```python
from build123d import *
from build123d.topology import SkipClean

# Parameters (mm, degrees)
BOSS_EXTRUDE1_DEPTH   = 20
CUT_EXTRUDE1_DEPTH    = 18.4
SKETCH3_W             = 14.5
SKETCH3_H             = 2.85
CUT_EXTRUDE2_DEPTH    = 18.4
SKETCH4_W             = 13
SKETCH4_H             = 1.4
BOSS_EXTRUDE2_DEPTH   = 22
BOSS_EXTRUDE2_2_DEPTH = 22
SKETCH5_W             = 13
SKETCH5_H             = 3.4
BOSS_EXTRUDE3_DEPTH   = 4
FILLET1_R             = 3.2
FILLET2_R             = 3.2
BOSS_EXTRUDE4_DEPTH   = 13
SKETCH8_W             = 0.8
SKETCH8_H             = 3.26
CUT_EXTRUDE3_DEPTH    = 13
FILLET3_R             = 3.2
FILLET4_R             = 0.8
SKETCH9_W             = 56.2
SKETCH9_H             = 1.6
BOSS_EXTRUDE5_DEPTH   = 10
SKETCH13_W            = 15.95
SKETCH13_H            = 1.6
CUT_EXTRUDE6_DEPTH    = 2
BOSS_EXTRUDE6_DEPTH   = 18.4
CUT_EXTRUDE5_START    = -18.4
SKETCH12_R            = 1.1
CUT_EXTRUDE5_DEPTH    = 18.4
SKETCH14_W            = 15.95
SKETCH14_H            = 5.75
CUT_EXTRUDE7_DEPTH    = 10


with BuildPart() as part:
    # Sketch1 → Boss-Extrude1 (new body)
    with BuildSketch(Plane(origin=(0, 0, 0), x_dir=(1, 0, 0), z_dir=(0, 1, 0))):
        Polygon((-38.4, 43.8), (-38.4, 40.4), (-21, 40.4), (-21, 43.8), (0, 43.8), (0, 0), (-21, 0), (-21, 3.4), (-38.4, 3.4), (-38.4, 0), (-59.4, 0), (-59.4, 43.8), align=None)
    extrude(amount=BOSS_EXTRUDE1_DEPTH)

    # Sketch2 → Cut-Extrude1 (cut)
    with BuildSketch(Plane(origin=(0, 20, 0), x_dir=(1, 0, 0), z_dir=(0, 1, 0))):
        Polygon((-57.8, 42.2), (-39.6, 42.2), (-39.6, 39.2), (-19.8, 39.2), (-19.8, 42.2), (-1.6, 42.2), (-1.6, 1.6), (-19.8, 1.6), (-19.8, 4.6), (-39.6, 4.6), (-39.6, 1.6), (-57.8, 1.6), align=None)
    extrude(amount=-CUT_EXTRUDE1_DEPTH, mode=Mode.SUBTRACT)

    # Sketch3 → Cut-Extrude2 (cut)
    with BuildSketch(Plane(origin=(0, 1.6, 0), x_dir=(1, 0, 0), z_dir=(0, 1, 0))):
        with Locations((-8.85, 37.875)):
            Rectangle(SKETCH3_W, SKETCH3_H)
    extrude(amount=-CUT_EXTRUDE2_DEPTH, mode=Mode.SUBTRACT)



with BuildPart() as body_2:
    # Sketch4 → Boss-Extrude2 (new body)
    with BuildSketch(Plane.XZ):
        with Locations((-29.7, -0.7)):
            Rectangle(SKETCH4_W, SKETCH4_H)
    extrude(amount=-BOSS_EXTRUDE2_DEPTH)


with BuildPart() as body_3:
    # Sketch4 → Boss-Extrude2 2 (new body)
    with BuildSketch(Plane.XZ):
        with Locations((-29.7, -43.1)):
            Rectangle(SKETCH4_W, SKETCH4_H)
    extrude(amount=-BOSS_EXTRUDE2_2_DEPTH)


with BuildPart() as part_1:
    add(part.part)

    add(body_2.part)  # Boss-Extrude3 merges body 2

    add(body_3.part)  # Boss-Extrude3 merges body 3
    # Sketch5 → Boss-Extrude3 (add)
    with BuildSketch(Plane(origin=(0, 0, 0), x_dir=(-1, 0, 0), z_dir=(0, -1, 0))):
        with Locations((29.7, 1.7)):
            Rectangle(SKETCH5_W, SKETCH5_H)
        with Locations((29.7, 42.1)):
            Rectangle(SKETCH5_W, SKETCH5_H)
    extrude(amount=-BOSS_EXTRUDE3_DEPTH)

    # Fillet1
    fillet1_edges = [part_1.edges().sort_by_distance(p)[0] for p in [
        (-29.7, 0, -43.8),
        (-29.7, 0, 0),
    ]]
    fillet(fillet1_edges, radius=FILLET1_R)

    # Fillet2
    # the kernel refuses this fillet: 3.2 mm, written as the material it adds along each edge
    with BuildSketch(Plane(origin=(-36.2, 4, -1.4), x_dir=(0, 0, -1), z_dir=(1, 0, 0)), Plane(origin=(-23.2, 4, -42.4), x_dir=(0, 0, 1), z_dir=(-1, 0, 0))) as fillet2_piece_1:
        with BuildLine():
            CenterArc((3.2, 2.966479395), FILLET2_R, 180, 67.975687163)
            Line((0, 2.966479395), (-0.064, 2.966479395))
            Line((-0.064, 2.966479395), (-0.064, 0))
            Line((-0.064, 0), (0, -0.064))
            ThreePointArc((0, -0.064), (1, -0.064), (1.976, -0.059329588))
            Line((1.976, -0.059329588), (2, 0))
        make_face()
    extrude(amount=13)

    # Sketch7 → Boss-Extrude4 (add)
    with BuildSketch(Plane(origin=(-23.2, 0, 0), x_dir=(0, 0, -1), z_dir=(1, 0, 0))):
        Polygon((-1.2, 17), (0, 17), (0, 11.8), align=None)
        Polygon((43.8, 11.8), (43.8, 17), (45, 17), align=None)
        Polygon((0, 22), (-3, 22), (-3, 20.26), (1.4, 20.26), (1.4, 22), (1.4, 26), (0, 26), align=None)
        Polygon((43.8, 22), (46.8, 22), (46.8, 20.26), (42.4, 20.26), (42.4, 22), (42.4, 26), (43.8, 26), align=None)
    extrude(amount=-BOSS_EXTRUDE4_DEPTH)

    # Sketch8 → Cut-Extrude3 (cut)
    with BuildSketch(Plane(origin=(-23.2, 0, 0), x_dir=(0, 0, -1), z_dir=(1, 0, 0))):
        with Locations((0.4, 18.63)):
            Rectangle(SKETCH8_W, SKETCH8_H)
        with Locations((43.4, 18.63)):
            Rectangle(SKETCH8_W, SKETCH8_H)
    extrude(amount=-CUT_EXTRUDE3_DEPTH, mode=Mode.SUBTRACT)

    # Fillet3
    # the kernel refuses this fillet: 3.2 mm, written as the material it adds along each edge
    with BuildSketch(Plane(origin=(-36.2, 22, 0), x_dir=(0, 1, 0), z_dir=(1, 0, 0)), Plane(origin=(-23.2, 22, -43.8), x_dir=(0, 1, 0), z_dir=(-1, 0, 0))) as fillet3_piece_1:
        with BuildLine():
            CenterArc((3.193743885, 3.2), FILLET3_R, 183.583321698, 86.416678302)
            Line((0, 3), (-0.063874878, 2.996))
            ThreePointArc((-0.063874878, 2.996), (-0.064, 1.5), (-0.064, 0))
            Line((-0.064, 0), (0, -0.064))
            Line((0, -0.064), (3.193743885, -0.064))
            Line((3.193743885, -0.064), (3.193743885, 0))
        make_face()
    extrude(amount=13)

    # Fillet4
    fillet4_edges = [part_1.edges().sort_by_distance(p)[0] for p in [
        (-29.7, 20.26, -0.8),
        (-29.7, 20.26, -43),
    ]]
    fillet(fillet4_edges, radius=FILLET4_R)

    # Sketch9 → Boss-Extrude5 (add)
    with BuildSketch(Plane(origin=(0, 1.6, 0), x_dir=(1, 0, 0), z_dir=(0, 1, 0))):
        Polygon((-57.8, 35), (-19.8, 35), (-19.8, 39.2), (-19.8, 42.2), (-1.6, 42.2), (-1.6, 40.75), (-17.55, 40.75), (-17.55, 35), (-1.6, 35), (-1.6, 33.4), (-57.8, 33.4), align=None)
        with Locations((-29.7, 9.6)):
            Rectangle(SKETCH9_W, SKETCH9_H)
    extrude(amount=BOSS_EXTRUDE5_DEPTH)

    # Sketch13 → Cut-Extrude6 (cut)
    with BuildSketch(Plane(origin=(0, 11.6, 0), x_dir=(1, 0, 0), z_dir=(0, 1, 0))):
        with Locations((-9.575, 34.2)):
            Rectangle(SKETCH13_W, SKETCH13_H)
    extrude(amount=-CUT_EXTRUDE6_DEPTH, mode=Mode.SUBTRACT)

    # Sketch11 → Boss-Extrude6 (add)
    with BuildSketch(Plane(origin=(0, 1.6, 0), x_dir=(1, 0, 0), z_dir=(0, 1, 0))):
        with BuildLine():
            Line((-57.8, 41.1), (-57.8, 40))
            ThreePointArc((-57.8, 40), (-56.244365081, 40.644365081), (-55.6, 42.2))
            Line((-55.6, 42.2), (-56.7, 42.2))
            ThreePointArc((-56.7, 42.2), (-57.022182541, 41.422182541), (-57.8, 41.1))
        make_face()
        with BuildLine():
            Line((-56.7, 1.6), (-55.6, 1.6))
            ThreePointArc((-55.6, 1.6), (-56.244365081, 3.155634919), (-57.8, 3.8))
            Line((-57.8, 3.8), (-57.8, 2.7))
            ThreePointArc((-57.8, 2.7), (-57.022182541, 2.377817459), (-56.7, 1.6))
        make_face()
        with BuildLine():
            Line((-1.6, 40), (-1.6, 41.1))
            ThreePointArc((-1.6, 41.1), (-2.377817459, 41.422182541), (-2.7, 42.2))
            Line((-2.7, 42.2), (-3.8, 42.2))
            ThreePointArc((-3.8, 42.2), (-3.155634919, 40.644365081), (-1.6, 40))
        make_face()
        with BuildLine():
            ThreePointArc((-1.6, 3.8), (-3.155634919, 3.155634919), (-3.8, 1.6))
            Line((-3.8, 1.6), (-1.6, 1.6))
            Line((-1.6, 1.6), (-1.6, 3.8))
        make_face()
    extrude(amount=BOSS_EXTRUDE6_DEPTH)

    # Sketch12 → Cut-Extrude5 (cut)
    with SkipClean():  # the faces are left unmerged after this step: merging them gives an invalid solid
        with BuildSketch(Plane(origin=(0, 20, 0), x_dir=(1, 0, 0), z_dir=(0, 1, 0)).offset(CUT_EXTRUDE5_START)):
            with Locations(Location((-57.8, 42.2, 0), (0, 0, 270))):
                Circle(SKETCH12_R)
            with Locations(Location((-57.8, 1.6, 0), (0, 0, 270))):
                Circle(SKETCH12_R)
            with Locations(Location((-1.6, 1.6, 0), (0, 0, 270))):
                Circle(SKETCH12_R)
            with Locations(Location((-1.6, 42.2, 0), (0, 0, 270))):
                Circle(SKETCH12_R)
        extrude(amount=CUT_EXTRUDE5_DEPTH, mode=Mode.SUBTRACT)

    # Sketch14 → Cut-Extrude7 (cut)
    with SkipClean():  # the faces are left unmerged after this step: merging them gives an invalid solid
        with BuildSketch(Plane(origin=(0, 1.6, 0), x_dir=(1, 0, 0), z_dir=(0, 1, 0))):
            with Locations((-9.575, 37.875)):
                Rectangle(SKETCH14_W, SKETCH14_H)
        extrude(amount=CUT_EXTRUDE7_DEPTH, mode=Mode.SUBTRACT)


solid = part_1.part
```
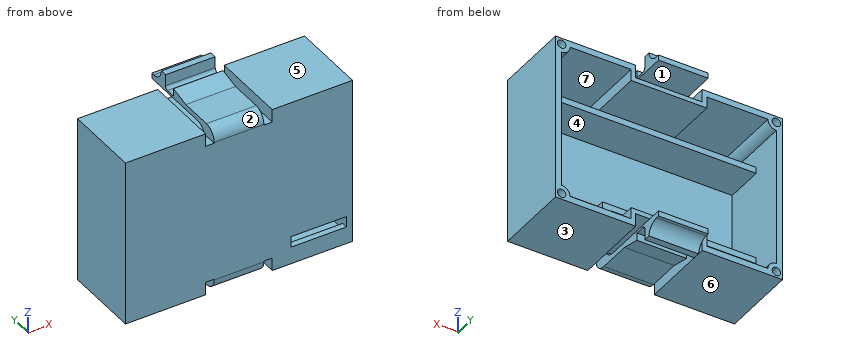
Source: CAD feature listing. Evaluate the final solid. Frame: model axes, mm. Face numbers are marked on the shaded views. A direction names the side the tool comes from. Coordinates: 2 decimals unless noted, no trailing zeros. Write each loop counter-clockwise with the first axis right and the second up, starting at its lowest first coordinate (ties: lowest second). Pieces come first, ordered by that corner, then holes. Notation, with made-up numbers: (7, 52) -> (28, 52) arc R14 cw to (28, 57) -> close; hole circle Ø4 at (41, 65.5). An arc over 180 degrees is marked (long way). Return JSON: item names as keys, results as strings. Group by question number.
1) Set-up query: the marked faces 1, 2 and 3. Return all of +Z, -Z, +X, -X, +Y, -Y with unobstructed straight access to the full face (end or side cutting, diameter ignored); none if empty.
2) Section query A-A, the plane x = -9.5. Return loops of the section in (y, z).
3) Contact query for flat-ended pins moving along their axis: P1, Ø2, axis at x = -57.8, z = -1.6, coming from the -Y side; P2, Ø10, axis at x = -43, y = 5, coming from the -Z side; P3, Ø1.8, axis at x = -27, z = -9.5, coming from the +Y side; P4, Ø0.8, axis at x = -11, y = 1, coming from the +Z side. Output: stop coordinate, or through.
4) Mould query, pull axis Z, two halves, no side actions, for the marked faces 4, 5, 6 and 7. Classes: +Z half, -Z half, draft (parallel to the pull), parting line (faces both ways), or undercut.
5) Ray query, line 1 along Z through (x, y) = (-16, 6); line 2 along Z through (x, y) = (-45.5, 6.5); line 3 along X through (y, z) = (9.5, -6). Return the intervals inside material, ascending.
6) Section query B-B, the plane z = -22.5. Return loops of the section in (x, y), plus the area to 3 significant figures.
From the geometry:
{
 "1": {"face 1": "+Y", "face 2": "+Z, -Y", "face 3": "-Z, +X, +Y, -Y"},
 "2": {"outline": "(0, -43.8) -> (20, -43.8) -> (20, -42.2) -> (11.6, -42.2) -> (11.6, -40.75) -> (1.6, -40.75) -> (1.6, -39.3) -> (0, -39.3) -> close; (0, -36.45) -> (1.6, -36.45) -> (1.6, -35) -> (9.6, -35) -> (9.6, -33.4) -> (1.6, -33.4) -> (1.6, -10.4) -> (11.6, -10.4) -> (11.6, -8.8) -> (1.6, -8.8) -> (1.6, -1.6) -> (20, -1.6) -> (20, 0) -> (0, 0) -> close"},
 "3": {"P1": "y = 0", "P2": "z = -43.8", "P3": "y = 11.6", "P4": "z = 0"},
 "4": {"face 4": "undercut", "face 5": "+Z half", "face 6": "-Z half", "face 7": "undercut"},
 "5": {"line 1": "-43.8 to -40.75, -35 to -33.4, -10.4 to -8.8, -1.6 to 0", "line 2": "-43.8 to -42.2, -35 to -33.4, -10.4 to -8.8, -1.6 to 0", "line 3": "-59.4 to -57.8, -1.6 to 0"},
 "6": {"outline": "(-59.4, 0) -> (0, 0) -> (0, 20) -> (-1.6, 20) -> (-1.6, 1.6) -> (-57.8, 1.6) -> (-57.8, 20) -> (-59.4, 20) -> close", "area": "154 mm²"}
}
